```python
from build123d import *

# Parameters (mm, degrees)
SKETCH1_W                                            = 72
SKETCH1_H                                            = 32.5
BOSS_EXTRUDE1_DEPTH                                  = 4
CBORE_FOR_M2_5_HEX_SOCKET_HEAD_CAP_SCREW_D           = 2.9
CBORE_FOR_M2_5_HEX_SOCKET_HEAD_CAP_SCREW_CBORE_D     = 5.5
CBORE_FOR_M2_5_HEX_SOCKET_HEAD_CAP_SCREW_CBORE_DEPTH = 2.9
SKETCH5_W                                            = 26
SKETCH5_H                                            = 2
BOSS_EXTRUDE2_DEPTH                                  = 15


with BuildPart() as part:
    # Sketch1 → Boss-Extrude1 (new body)
    with BuildSketch(Plane(origin=(0, 0, 0), x_dir=(1, 0, 0), z_dir=(0, 1, 0))):
        with Locations((36, 16.25)):
            Rectangle(SKETCH1_W, SKETCH1_H)
    extrude(amount=BOSS_EXTRUDE1_DEPTH)

    # CBORE for M2.5 Hex Socket Head Cap Screw1 (through all)
    with Locations(Plane(origin=(0, 4, 0), x_dir=(1, 0, 0), z_dir=(0, 1, 0))):
        with Locations((-10.4, 24.25), (1.6, 24.25), (1.6, 8.25), (-10.4, 8.25), (82.4, 8.25), (70.4, 8.25), (70.4, 24.25), (82.4, 24.25)):
            CounterBoreHole(CBORE_FOR_M2_5_HEX_SOCKET_HEAD_CAP_SCREW_D / 2, CBORE_FOR_M2_5_HEX_SOCKET_HEAD_CAP_SCREW_CBORE_D / 2, CBORE_FOR_M2_5_HEX_SOCKET_HEAD_CAP_SCREW_CBORE_DEPTH)

    # Sketch5 → Boss-Extrude2 (add)
    with BuildSketch(Plane.XZ):
        with Locations((13, -1)):
            Rectangle(SKETCH5_W, SKETCH5_H)
        with Locations((13, -31.5)):
            Rectangle(SKETCH5_W, SKETCH5_H)
        with Locations((59, -1)):
            Rectangle(SKETCH5_W, SKETCH5_H)
        with Locations((59, -31.5)):
            Rectangle(SKETCH5_W, SKETCH5_H)
    extrude(amount=BOSS_EXTRUDE2_DEPTH)


solid = part.part
```
Can you work these out from the model? Positions are in its coordinate system, mm. A direction names the side the tool comes from. Give positions to 0.01 mm unless a question says otherwise; leave off trailing zeros. Loops run counter-clockwise (first coordinate to the right, second up) from the corner with the lowest first, then second, coordinate; pieces in that order, holes last. Notation, with made-up numbers: M -23.5,-25 L 31.5,-25 A16 cw 31.5,-2 Z; hole C 78,-36 d2. An arc over 180 degrees is marked long. Use CSV: the item, a comma, the result in double quotes. Start each with the question number.
1. Imagine slicing it at C-C, the plane z = -24.25. Write out the boundary of the cut face in (x, y).
2. If we mould it in two halves opening along X, with no side actions, what happens to faces 1 (the face through (1.914, 0.542, -22.834)), 2 (the face through (72, 1, -15)), 3 (the face through (13, -7, -2))? For each: released by +X, released by -X, zero draft, split by the parting line, or undercut.
3. For P1, Ø16, axis at x = 44, z = -21, coming from the -Y side; P2, Ø3.5, axis at x = 1.6, z = -8.25, coming from the +Y side; P3, Ø2.5, axis at x = 1.6, z = -24.25, coming from the +Y side, each with a flat end and sliding along its axis, tell me the tip position at first contact or that it passes through.
4. If I drill on L1, parallel to Z at x = 1.6, y = 0.5; L2, parallel to X at y = 0.75, z = -8.25; L3, parallel to Z at x = 68.5, y = -1.75, over which ranges is the centre line in solid material (lowest first)?
5. Imagine slicing it at A-A, the plane y = -8.75. Write out the boundary of the cut face in (x, z).
6. Imagine slicing it at D-D, the plane x = 13. Write out the boundary of the cut face in (y, z), plus the area to 3 significant figures.
7. Imagine slicing it at B-B, the plane x = 1.6. Write out the boundary of the cut face in (y, z), plus the area to 3 significant figures.
8. On a 3-axis mill with a long thin cutter (end or side, diameter ignored), from which of +Z, -Z, +X, -X, +Y, -Y can I reach the whole of each face in a straight line? I mean faces 4 (the face through (3.11, 1.1, -23.68)), 5 (the face through (59, -7, -2)), 6 (the face through (46, -7, -32)). Say none if no direction works.
Response values:
1,outline,"M 0,0 L 0.15,0 L 0.15,1.1 L 0,1.1 Z; M 3.05,0 L 68.95,0 L 68.95,1.1 L 67.65,1.1 L 67.65,4 L 4.35,4 L 4.35,1.1 L 3.05,1.1 Z; M 71.85,0 L 72,0 L 72,1.1 L 71.85,1.1 Z"
2,face 1,"undercut"
2,face 2,"released by +X"
2,face 3,"zero draft"
3,P1,"y = 0"
3,P2,"y = 1.1"
3,P3,"through"
4,L1,"-32.5 to -25.7, -22.8 to -9.7, -6.8 to 0"
4,L2,"0 to 0.15, 3.05 to 68.95, 71.85 to 72"
4,L3,"-32.5 to -30.5, -2 to 0"
5,outline,"M 0,-32.5 L 26,-32.5 L 26,-30.5 L 0,-30.5 Z; M 0,-2 L 26,-2 L 26,0 L 0,0 Z; M 46,-32.5 L 72,-32.5 L 72,-30.5 L 46,-30.5 Z; M 46,-2 L 72,-2 L 72,0 L 46,0 Z"
6,outline,"M -15,-32.5 L 4,-32.5 L 4,0 L -15,0 L -15,-2 L 0,-2 L 0,-30.5 L -15,-30.5 Z"
6,area,"190 mm^2"
7,outline,"M -15,-32.5 L 4,-32.5 L 4,-27 L 1.1,-27 L 1.1,-25.7 L 0,-25.7 L 0,-30.5 L -15,-30.5 Z; M -15,-2 L 0,-2 L 0,-6.8 L 1.1,-6.8 L 1.1,-5.5 L 4,-5.5 L 4,0 L -15,0 Z; M 0,-22.8 L 1.1,-22.8 L 1.1,-21.5 L 4,-21.5 L 4,-11 L 1.1,-11 L 1.1,-9.7 L 0,-9.7 Z"
7,area,"152 mm^2"
8,face 4,"+Y"
8,face 5,"+X, -X, -Y"
8,face 6,"+Z, -Z, -Y"
